Read the model definition and answer for the solid it produces. Units are mm, in the model's axes. Give positions to 0.01 mm unless a question says otherwise; leave off trailing zeros. Write each loop counter-clockwise with the first axis right and the second up, starting at its lowest first coordinate (ties: lowest second). Pieces come first, ordered by that corner, then holes. Notation, with made-up numbers: (87.25, -32.75) -> (132.25, -32.75) arc R24 ccw to (132.25, -4.75) -> close; hole circle Ø11 at (-34, 81). An arc over 180 degrees is marked (long way). Write item = value, one per line.
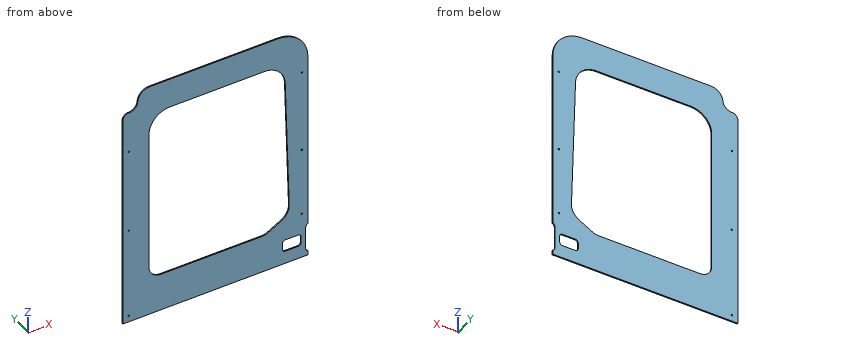
from build123d import *

# Parameters (mm, degrees)
F0_W      = 787.4
F0_H      = 1016
F1_DEPTH  = 5.08
F3_DEPTH  = 5.081
F5_DEPTH  = 5.081
F7_DEPTH  = 5.081
F9_DEPTH  = 5.081
F11_DEPTH = 5.081
F12_DEPTH = 25.4
F14_DEPTH = 5.081
F16_DEPTH = 5.081
F17_R     = 3.175
F18_DEPTH = 5.081


with BuildPart() as f1:
    # F0 (on Front) → F1 (new body)
    with BuildSketch(Plane.XZ):
        with Locations((0.161311, 159.993043)):
            Rectangle(F0_W, F0_H)
    extrude(amount=F1_DEPTH)

    # F2 (on face) → F3 (cut, through all)
    with BuildSketch(Plane.XZ.offset(5.08)):
        with BuildLine():
            Line((352.586311, -243.231957), (298.611311, -243.231957))
            ThreePointArc((298.611311, -243.231957), (289.631055, -246.951701), (285.911311, -255.931957))
            Line((285.911311, -255.931957), (285.911311, -281.331957))
            ThreePointArc((285.911311, -281.331957), (289.631055, -290.312213), (298.611311, -294.031957))
            Line((298.611311, -294.031957), (352.586311, -294.031957))
            ThreePointArc((352.586311, -294.031957), (361.566567, -290.312213), (365.286311, -281.331957))
            Line((365.286311, -281.331957), (365.286311, -255.931957))
            ThreePointArc((365.286311, -255.931957), (361.566567, -246.951701), (352.586311, -243.231957))
        make_face()
    extrude(amount=-F3_DEPTH, mode=Mode.SUBTRACT)

    # F4 (on face) → F5 (cut, through all)
    with BuildSketch(Plane.XZ.offset(5.08)):
        with BuildLine():
            ThreePointArc((403.386311, -205.131957), (389.915926, -210.711573), (384.336311, -224.181957))
            Line((384.336311, -224.181957), (384.336311, -313.081957))
            ThreePointArc((384.336311, -313.081957), (389.915926, -326.552341), (403.386311, -332.131957))
            Line((403.386311, -332.131957), (403.386311, -205.131957))
        make_face()
    extrude(amount=-F5_DEPTH, mode=Mode.SUBTRACT)

    # F6 (on face) → F7 (cut, through all)
    with BuildSketch(Plane.XZ.offset(5.08)):
        with BuildLine():
            Line((208.69992, 544.168043), (-193.513689, 544.168043))
            ThreePointArc((-193.513689, 544.168043), (-256.375482, 518.129836), (-282.413689, 455.268043))
            Line((-282.413689, 455.268043), (-282.413689, -138.456957))
            ThreePointArc((-282.413689, -138.456957), (-267.534714, -174.377981), (-231.613689, -189.256957))
            Line((-231.613689, -189.256957), (196.694191, -189.256957))
            ThreePointArc((196.694191, -189.256957), (212.384245, -187.288024), (227.101301, -181.503326))
            Line((227.101301, -181.503326), (281.64154, -151.754104))
            ThreePointArc((281.64154, -151.754104), (306.334633, -127.570652), (314.703824, -94.036418))
            Line((314.703824, -94.036418), (297.557071, 458.027888))
            ThreePointArc((297.557071, 458.027888), (270.578268, 519.098131), (208.69992, 544.168043))
        make_face()
    extrude(amount=-F7_DEPTH, mode=Mode.SUBTRACT)

    # F8 (on face) → F9 (cut, through all)
    with BuildSketch(Plane.XZ.offset(5.08)):
        with BuildLine():
            Line((-330.038689, 667.993043), (-393.538689, 667.993043))
            Line((-393.538689, 667.993043), (-393.538689, 585.443043))
            Line((-393.538689, 585.443043), (-368.138689, 585.443043))
            ThreePointArc((-368.138689, 585.443043), (-341.197921, 596.602275), (-330.038689, 623.543043))
            Line((-330.038689, 623.543043), (-330.038689, 667.993043))
        make_face()
    extrude(amount=-F9_DEPTH, mode=Mode.SUBTRACT)

    # F10 (on face) → F11 (cut, through all)
    with BuildSketch(Plane.XZ.offset(5.08)):
        with BuildLine():
            ThreePointArc((-330.038689, 617.193043), (-315.159714, 653.114068), (-279.238689, 667.993043))
            Line((-279.238689, 667.993043), (-330.038689, 667.993043))
            Line((-330.038689, 667.993043), (-330.038689, 617.193043))
        make_face()
    extrude(amount=-F11_DEPTH, mode=Mode.SUBTRACT)

    # F10 (on face) → F12 (cut)
    with BuildSketch(Plane.XZ.offset(5.08)):
        with BuildLine():
            ThreePointArc((-330.038689, 617.193043), (-315.159714, 653.114068), (-279.238689, 667.993043))
            Line((-279.238689, 667.993043), (-330.038689, 667.993043))
            Line((-330.038689, 667.993043), (-330.038689, 617.193043))
        make_face()
    extrude(amount=-F12_DEPTH, mode=Mode.SUBTRACT)

    # F13 (on face) → F14 (cut, through all)
    with BuildSketch(Plane.XZ.offset(5.08)):
        with BuildLine():
            ThreePointArc((-393.538689, 560.043043), (-386.099202, 578.003555), (-368.138689, 585.443043))
            Line((-368.138689, 585.443043), (-393.538689, 585.443043))
            Line((-393.538689, 585.443043), (-393.538689, 560.043043))
        make_face()
    extrude(amount=-F14_DEPTH, mode=Mode.SUBTRACT)

    # F15 (on face) → F16 (cut, through all)
    with BuildSketch(Plane.XZ.offset(5.08)):
        with BuildLine():
            ThreePointArc((266.861311, 667.993043), (356.663872, 630.795604), (393.861311, 540.993043))
            Line((393.861311, 540.993043), (393.861311, 667.993043))
            Line((393.861311, 667.993043), (266.861311, 667.993043))
        make_face()
    extrude(amount=-F16_DEPTH, mode=Mode.SUBTRACT)

    # F17 (on face) → F18 (cut, through all)
    with BuildSketch(Plane.XZ.offset(5.08)):
        with Locations((368.461311, 477.493043)):
            Circle(F17_R)
        with Locations((368.461311, 131.418043)):
            Circle(F17_R)
        with Locations((368.461311, -154.331957)):
            Circle(F17_R)
        with Locations((-368.138689, -321.019457)):
            Circle(F17_R)
        with Locations((-368.138689, 59.980543)):
            Circle(F17_R)
        with Locations((-368.138689, 412.405543)):
            Circle(F17_R)
    extrude(amount=-F18_DEPTH, mode=Mode.SUBTRACT)


solid = f1.part
(1) The part is cut by section C-C on y = -1. Count the separate pieces of the cut face and the enclosed holes in it, plus the area to 3 significant figures.
Checks:
separate_pieces = 1
enclosed_holes = 8
area = 361,000 mm²
(2) Consider L1, parallel to X at y = -1.55, z = -265.5; L2, parallel to Z at x = -151, y = -2.1; L3, parallel to X at y = -0.2, z = 456. Determine where each line is inside the solid, lowest interval first.
Checks:
L1 = -393.54 to 285.91, 365.29 to 384.34
L2 = -348.01 to -189.26, 544.17 to 667.99
L3 = -393.54 to -282.41, 297.62 to 393.86
(3) Given P1, Ø7.5, axis at x = 368.46, z = 477.49, coming from the +Y side; P2, Ø1.5, axis at y = -3, z = -263.5, coming from the +X side; P3, Ø2.5, axis at x = 313.5, y = -2.5, coming from the +Z side, each flat-ended and moving along its own axis, determine where each tip first touches the part or whether it passes through.
Checks:
P1 = 0
P2 = 384.34
P3 = 659.61
(4) The part is cut by section B-B on z = 170.5. Determine the outline of the cut face in (x, y), plus the area to 3 significant figures.
Checks:
outline = (-393.54, -5.08) -> (-282.41, -5.08) -> (-282.41, 0) -> (-393.54, 0) -> close; (306.49, -5.08) -> (393.86, -5.08) -> (393.86, 0) -> (306.49, 0) -> close
area = 1,010 mm²
(5) The part is cut by section A-A on x = -157.5. Determine the outline of the cut face in (y, z).
Checks:
outline = (-5.08, -348.01) -> (0, -348.01) -> (0, -189.26) -> (-5.08, -189.26) -> close; (-5.08, 544.17) -> (0, 544.17) -> (0, 667.99) -> (-5.08, 667.99) -> close
